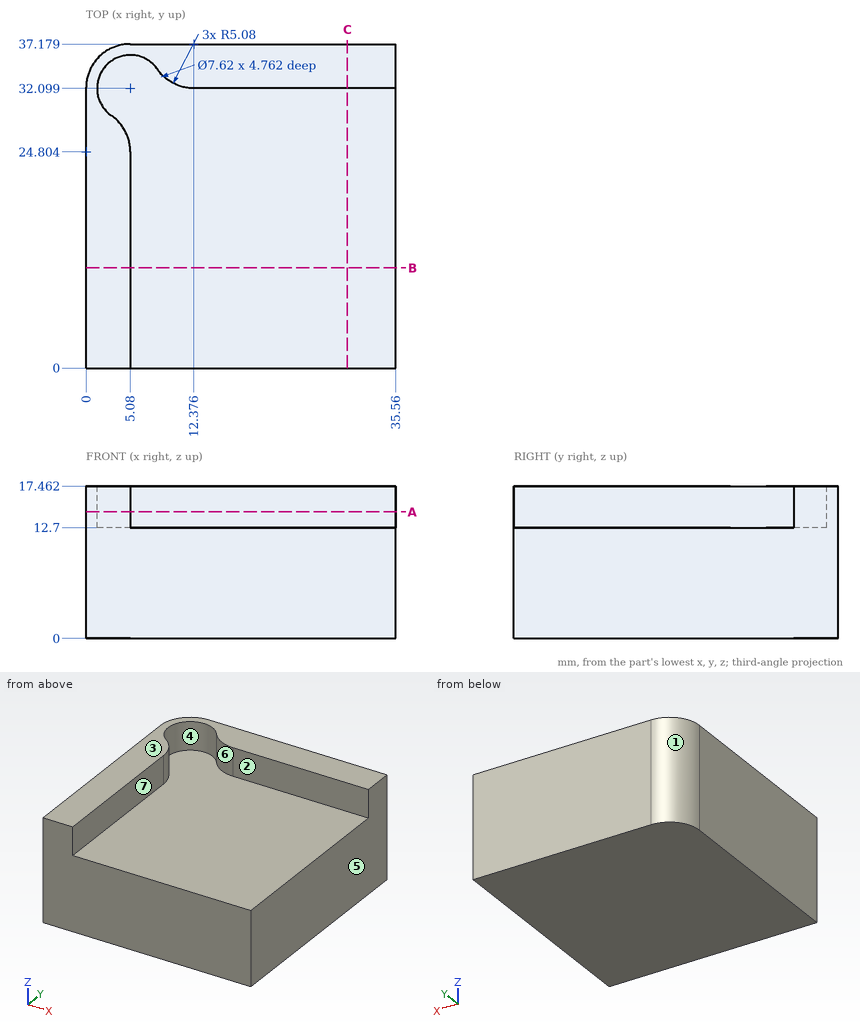
Verification items for this drawing (mm, ordinates from the low corner). A direction names the side the tool comes from. Give positions to 0.01 mm unless a question says otherwise; leave off trailing zeros. Order: outer loops, then holes, each group sorted by start corner. A loop starts at its lowest first (then second) coordinate and runs counter-clockwise, first axis right, second up. Notation, with made-up numbers: M -2.75,52 L 6.25,52 A24 ccw 6.25,62 Z; hole C 12.25,64.25 d4. An arc over 180 degrees is marked long. Use a Markdown table: item, result.
Item 1: Depth check by flat-ended pin: P1, Ø10.5, axis at x = 10, y = 15.5, coming from the +Z side; P2, Ø2.5, axis at x = 18, z = 16, coming from the -Y side; P3, Ø1.4, axis at y = 11, z = 14, coming from the +X side; P4, Ø6, axis at x = 31, y = 20, coming from the +Z side. Enter the tip coordinate at first touch or a pass-through.
Answers follow:
| item | result |
|---|---|
| P1 | stops at z = 17.46 |
| P2 | stops at y = 32.1 |
| P3 | stops at x = 5.08 |
| P4 | stops at z = 12.7 |
Item 2: Tool access check on the marked faces 5, 6 and 7. Record the directions out of +Z, -Z, +X, -X, +Y, -Y that give a thin tool (end or side, any length) a straight path to the whole face; none if there is none.
Answers follow:
| item | result |
|---|---|
| face 5 | +Z, -Z, +X, +Y, -Y |
| face 6 | +Z, -Y |
| face 7 | +Z, +X, -Y |
Item 3: Section check B-B (y = 11.5). Record the cut outline in (x, z), and give its area (3 significant figures).
Answers follow:
| item | result |
|---|---|
| outline | M 0,0 L 35.56,0 L 35.56,12.7 L 5.08,12.7 L 5.08,17.46 L 0,17.46 Z |
| area | 476 mm2 |
Item 4: Section check A-A (z = 14.5). Record the cut outline in (x, y) (1 decimal).
Answers follow:
| item | result |
|---|---|
| outline | M 0,0 L 5.1,0 L 5.1,24.8 A5.1 ccw 2.9,29 A3.8 cw long 8.2,34.3 A5.1 ccw 12.4,32.1 L 35.6,32.1 L 35.6,37.2 L 5.1,37.2 A5.1 ccw 0,32.1 Z |
Item 5: Draft check along Y on the marked faces 1, 2, 3 and 4. Enter one of: +Y half, -Y half, draft (parallel to the pull), parting line (faces both ways), or undercut.
Answers follow:
| item | result |
|---|---|
| face 1 | +Y half |
| face 2 | -Y half |
| face 3 | draft |
| face 4 | undercut |
Item 6: Section check C-C (x = 30). Record the cut outline in (y, z).
Answers follow:
| item | result |
|---|---|
| outline | M 0,0 L 37.18,0 L 37.18,17.46 L 32.1,17.46 L 32.1,12.7 L 0,12.7 Z |
Item 7: Material ranges on line 1 along Y through (x, z) = (5, 3.5); line 2 along Z through (x, y) = (10, 4.5); line 3 along X through (y, z) = (3.5, 14.25), recorded low to high.
Answers follow:
| item | result |
|---|---|
| line 1 | y = 0 to 37.18 |
| line 2 | z = 0 to 12.7 |
| line 3 | x = 0 to 5.08 |
